from build123d import *

# Parameters (mm, degrees)
EXTRUDE_1_DEPTH     = 10
SKETCH_2_R          = 1.7
CUT_EXTRUDE_1_DEPTH = 90
SKETCH_3_R          = 3.7
CUT_EXTRUDE_2_DEPTH = 43
FILLET_1_R          = 40


with BuildPart() as part:
    # 草图1 → 凸台-拉伸1 (new body)
    with BuildSketch(Plane(origin=(0, 0, 0), x_dir=(1, 0, 0), z_dir=(0, 1, 0))):
        with BuildLine():
            Line((28.65, -40), (44.5, -40))
            Line((44.5, -40), (44.5, 35))
            Line((44.5, 35), (-44.5, 35))
            Line((-44.5, 35), (-44.5, -40))
            Line((-44.5, -40), (-28.65, -40))
            Line((-28.65, -40), (-28.65, 0))
            ThreePointArc((-28.65, 0), (0, 28.65), (28.65, 0))
            Line((28.65, 0), (28.65, -40))
        make_face()
    extrude(amount=EXTRUDE_1_DEPTH)

    # 草图2 → 切除-拉伸1 (cut)
    with BuildSketch(Plane.XY.offset(40)):
        with Locations((-40, 5)):
            Circle(SKETCH_2_R)
        with Locations((40, 5)):
            Circle(SKETCH_2_R)
    extrude(amount=-CUT_EXTRUDE_1_DEPTH, mode=Mode.SUBTRACT)

    # 草图3 → 切除-拉伸2 (cut)
    with BuildSketch(Plane(origin=(0, 0, -35), x_dir=(-1, 0, 0), z_dir=(0, 0, -1))):
        with Locations((40, 5)):
            Circle(SKETCH_3_R)
        with Locations((-39.998802569, 5)):
            Circle(SKETCH_3_R)
    extrude(amount=-CUT_EXTRUDE_2_DEPTH, mode=Mode.SUBTRACT)

    # 圆角1
    # the kernel refuses this fillet: 40 mm, written as the material it takes off along each edge
    with BuildSketch(Plane(origin=(-44.5, -100, -35), x_dir=(1, 0, 0), z_dir=(0, 1, 0)), Plane(origin=(44.5, -100, -35), x_dir=(0, 0, 1), z_dir=(0, 1, 0))) as fillet_1_piece_1:
        with BuildLine():
            CenterArc((FILLET_1_R, -FILLET_1_R), FILLET_1_R, 90, 90)
            Line((0, -FILLET_1_R), (0, 0))
            Line((0, 0), (FILLET_1_R, 0))
        make_face()
    extrude(amount=210, mode=Mode.SUBTRACT)


solid = part.part
Model file for the job. Use its own axes, mm. A direction names the side the tool comes from. Give positions to 0.01 mm unless a question says otherwise; leave off trailing zeros. Write each loop counter-clockwise with the first axis right and the second up, starting at its lowest first coordinate (ties: lowest second). Pieces come first, ordered by that corner, then holes. Notation, with made-up numbers: (87, -31.75) - (132, -31.75) arc R21 cw to (132, -12.75) - close; hole circle Ø10 at (80, -21.75). An arc over 180 degrees is marked (long way). Answer as CSV lines item,"result".
1. Drill centre lines: L1, parallel to X at y = 6, z = 24.5; L2, parallel to Y at x = 40, z = 16.5; L3, parallel to X at y = 5, z = -25.5. Where is each one in solid material? Low to high. Write a range as [from, to].
Responses:
L1,"x = [-44.5, -41.37], [-38.63, -28.65], [28.65, 38.63], [41.37, 44.5]"
L2,"y = [0, 3.3], [6.7, 10]"
L3,"x = [-30.38, -13.06], [13.06, 30.38]"
2. Band-saw the part on D-D (z = -12). Write the cut outline in (x, y), and give its area (3 significant figures).
Responses:
outline,"(-40.71, 0) - (-26.02, 0) - (-26.02, 10) - (-40.71, 10) - (-40.71, 8.63) arc R3.7 cw (long way) to (-40.71, 1.37) - close; (26.02, 0) - (40.71, 0) - (40.71, 1.37) arc R3.7 cw (long way) to (40.71, 8.63) - (40.71, 10) - (26.02, 10) - close"
area,"240 mm2"
3. Pin check, flat tips, straight feed: pin 1 (6 mm diameter, centred on y = 1.5, z = 0, fed in from +X); pin 2 (4.5 mm diameter, centred on x = 40, y = 5, fed in from -Z); pin 3 (1 mm diameter, centred on x = -24, y = 4, fed in from +Z). Stop position of each tip, or through.
Responses:
pin 1,"stops at x = 44.45"
pin 2,"stops at z = 8"
pin 3,"stops at z = -14.85"
4. Band-saw the part on A-A (z = 30). Write the cut outline in (x, y).
Responses:
outline,"(-44.5, 0) - (-28.65, 0) - (-28.65, 10) - (-44.5, 10) - close; (28.65, 0) - (44.5, 0) - (44.5, 10) - (28.65, 10) - close; hole circle Ø3.4 at (-40, 5); hole circle Ø3.4 at (40, 5)"
5. Band-saw the part on C-C (y = 2.25). Write the cut outline in (x, z).
Responses:
outline,"(-44.5, 5) arc R40 ccw to (-42.48, -7.56) - (-42.48, 8) - (-37.52, 8) - (-37.52, -17.57) arc R40 ccw to (-4.5, -35) - (4.5, -35) arc R40 ccw to (37.52, -17.57) - (37.52, 8) - (42.47, 8) - (42.47, -7.57) arc R40 ccw to (44.5, 5) - (44.5, 40) - (28.65, 40) - (28.65, 0) arc R28.65 cw to (-28.65, 0) - (-28.65, 40) - (-44.5, 40) - close"
6. Band-saw the part on B-B (x = 40). Write the cut outline in (y, z), and give its area (3 significant figures).
Responses:
outline,"(0, -13.43) - (1.3, -13.43) - (1.3, 8) - (3.3, 8) - (3.3, 40) - (0, 40) - close; (6.7, 8) - (8.7, 8) - (8.7, -13.43) - (10, -13.43) - (10, 40) - (6.7, 40) - close"
area,"267 mm2"
7. Two-plate mould, pull along Y, no slides. Class faces 4 (the face through (29, 10, 2)), 5 (the face through (-36.304, 5.163, -2.794)), 6 (the face through (-0.63, 4.93, -28.643)): +Y half, -Y half, draft (parallel to the pull), parting line (faces both ways), or undercut.
Responses:
face 4,"+Y half"
face 5,"undercut"
face 6,"draft"
8. 3-axis set-ups, long thin cutter, end or side, ignore diameter. For faces 1 (the face through (38, 4, 8)), 2 (the face through (28.65, 5, 20)), 3 (the face through (-37, 5, 40)): which of +Z, -Z, +X, -X, +Y, -Y reach the whole face in a straight line?
Responses:
face 1,"-Z"
face 2,"+Z, +Y, -Y"
face 3,"+Z, +X, -X, +Y, -Y"
